The drawing under review shows one solid part. Ordinate dimensions are in mm from its lowest x, y, z. A direction names the side the tool comes from. Round coordinates to 2 decimals unless told otherwise and drop trailing zeros. Loops run counter-clockwise (first coordinate to the right, second up) from the corner with the lowest first, then second, coordinate; pieces in that order, holes last. Notation, with made-up numbers: (-5, -12.5) -> (36, -12.5) arc R6 ccw to (36, -6.5) -> close; hole circle Ø10 at (72, 34). An arc over 180 degrees is marked (long way). Answer as CSV lines item,"result". Start each with the question number.
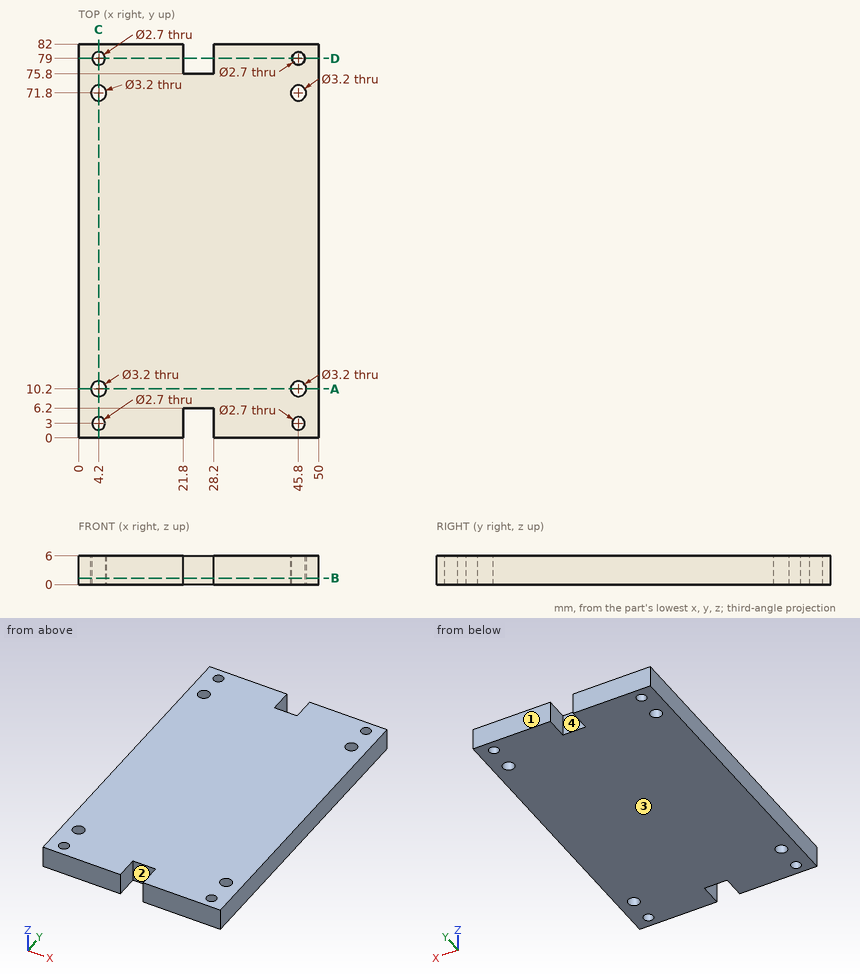
Q1. For pin 1 Ø1 at (x, y) = (8, 62) entering from -Z; pin 2 Ø1.9 at (x, y) = (45.8, 71.8) entering from +Z, all flat-tipped, find the tip position at first contact; note any pin that passes through.
Q2. Add section C-C, the plane x = 4.2. Give the boundary of the cut face in (y, z).
Q3. Add section B-B, the plane z = 1.35. State how many separate pieces and enclosed holes the cut face has, and give its area (3 significant figures).
Q4. Mouldability with a two-part tool opening along X and no side actions: class the marked faces 1 and 2 as pulls with the +X half, pulls with the -X half, needs draft (parallel to the pull), parting line crosses it, or undercut.
Q5. Machinability: for the marked faces 3 and 4, which of the approach directions +Z, -Z, +X, -X, +Y, -Y give a long, thin tool a straight path to every point of the face, cutting with its end or side? Answer none if there is none.
Q6. Add section D-D, the plane y = 79. Give the boundary of the cut face in (x, z), and give its area (3 significant figures).
Q7. To check wall thickness, follow probe 1 along Y at (x, z) = (45.8, 2.65); probe 2 along X at (y, z) = (79, 1.6); probe 3 along X at (y, z) = (71.8, 2.5). State the ranges of each line that lie inside material, in increasing order. Write a range as from..to.
Q8. Add section A-A, the plane y = 10.2. Give the boundary of the cut face in (x, z), and give its area (3 significant figures).
Worked answers:
1,pin 1,"stops at z = 0"
1,pin 2,"passes through"
2,outline,"(0, 0) -> (1.65, 0) -> (1.65, 6) -> (0, 6) -> close; (4.35, 0) -> (8.6, 0) -> (8.6, 6) -> (4.35, 6) -> close; (11.8, 0) -> (70.2, 0) -> (70.2, 6) -> (11.8, 6) -> close; (73.4, 0) -> (77.65, 0) -> (77.65, 6) -> (73.4, 6) -> close; (80.35, 0) -> (82, 0) -> (82, 6) -> (80.35, 6) -> close"
3,separate pieces,"1"
3,enclosed holes,"8"
3,area,"3,970 mm^2"
4,face 1,"needs draft"
4,face 2,"undercut"
5,face 3,"-Z, +X, -X, +Y, -Y"
5,face 4,"+Z, -Z, +Y"
6,outline,"(0, 0) -> (2.85, 0) -> (2.85, 6) -> (0, 6) -> close; (5.55, 0) -> (21.8, 0) -> (21.8, 6) -> (5.55, 6) -> close; (28.2, 0) -> (44.45, 0) -> (44.45, 6) -> (28.2, 6) -> close; (47.15, 0) -> (50, 0) -> (50, 6) -> (47.15, 6) -> close"
6,area,"229 mm^2"
7,probe 1,"y = 0..1.65, 4.35..8.6, 11.8..70.2, 73.4..77.65, 80.35..82"
7,probe 2,"x = 0..2.85, 5.55..21.8, 28.2..44.45, 47.15..50"
7,probe 3,"x = 0..2.6, 5.8..44.2, 47.4..50"
8,outline,"(0, 0) -> (2.6, 0) -> (2.6, 6) -> (0, 6) -> close; (5.8, 0) -> (44.2, 0) -> (44.2, 6) -> (5.8, 6) -> close; (47.4, 0) -> (50, 0) -> (50, 6) -> (47.4, 6) -> close"
8,area,"262 mm^2"
